Autodesk Fusion 360 part; units mm, degrees
sketch "Sketch1" plane through (0, 0, 0) normal (0, 0, 1) x (1, 0, 0)
  line L0 (0, 0) -> (-89.8767, -4.7102)
  line L1 (0, 0) -> (90, 0) construction
  line L2 (0, 0) -> (0, 36)
  line L3 (0, 36) -> (-89.8767, 40.7102)
  line L4 (0, 36) -> (90, 36) construction
  line L5 (-89.8767, 40.7102) -> (-89.8767, -4.7102)
  dimension "d1" = 177
  dimension "d2" = 90
  dimension "d3" = 36
  dimension "d4" = 177
  dimension "d5" = 90
extrude "Extrude1" add sketch "Sketch1" along normal blind 6 draft 45
fillet "Fillet1" radius 10 2 edges at (3, -2.8469, 3) (3, 38.8469, 3)
sketch "Sketch2" plane through (0, 0, 0) normal (0, 0, -1) x (1, 0, 0)
  ellipse E0 centre (-14.1421, -22.5796) end of major axis (-1.7883, -34.3029) minor radius 10 (-6.701, -36.3512) -> (0, -29.2898) ccw
  line L0 (0, -29.2898) -> (0, -6.7102)
  ellipse E1 centre (-14.1421, -13.4204) end of major axis (-1.7883, -1.6971) minor radius 10 (0, -6.7102) -> (-6.701, 0.3512) ccw
  line L1 (-6.701, 0.3512) -> (-89.8767, 4.7102)
  line L2 (-89.8767, 4.7102) -> (-89.8767, -40.7102)
  line L3 (-89.8767, -40.7102) -> (-6.701, -36.3512)
  line L4 (-89.8767, 4.7102) -> (-89.8767, -18) construction
  line L5 (-89.8767, -18) -> (-45.8767, -18) construction
  line L6 (-6.8767, -33.25) -> (-84.8767, -33.25)
  line L7 (-84.8767, -33.25) -> (-84.8767, -2.75)
  line L8 (-84.8767, -2.75) -> (-6.8767, -2.75)
  line L9 (-6.8767, -2.75) -> (-6.8767, -33.25)
  line L10 (-6.8767, -33.25) -> (-84.8767, -2.75) construction
  line L11 (-84.8767, -33.25) -> (-6.8767, -2.75) construction
  point P0 (-45.8767, -18)
  dimension "d10" = 22.7102
  dimension "d11" = 44
  dimension "d12" = 78
  dimension "d13" = 30.5
extrude "Extrude2" cut sketch "Sketch2" against normal blind 1.5 contours L6 L7 L8 L9
sketch "Sketch3" plane through (0, 0, 0) normal (0, 0, -1) x (1, 0, 0)
  line L0 (-84.8767, -33.25) -> (-84.8767, -2.75)
  line L1 (-84.8767, -2.75) -> (-6.8767, -2.75)
  line L2 (-6.8767, -2.75) -> (-6.8767, -33.25)
  line L3 (-6.8767, -33.25) -> (-84.8767, -33.25)
  ellipse E0 centre (-14.1421, -22.5796) end of major axis (-1.7883, -34.3029) minor radius 10 (-6.701, -36.3512) -> (0, -29.2898) ccw
  line L4 (0, -29.2898) -> (0, -6.7102)
  ellipse E1 centre (-14.1421, -13.4204) end of major axis (-1.7883, -1.6971) minor radius 10 (0, -6.7102) -> (-6.701, 0.3512) ccw
  line L5 (-6.701, 0.3512) -> (-89.8767, 4.7102)
  line L6 (-89.8767, 4.7102) -> (-89.8767, -40.7102)
  line L7 (-89.8767, -40.7102) -> (-6.701, -36.3512)
sketch "Sketch4" plane through (0, 0, 0) normal (0, 0, -1) x (1, 0, 0)
  line L0 (-85, -15) -> (-85, 16.158)
  line L1 (-85, 16.158) -> (-101.3363, 16.158)
  line L2 (-101.3363, 16.158) -> (-101.3363, -48.0286)
  line L3 (-101.3363, -48.0286) -> (-85, -48.0286)
  line L4 (-85, -48.0286) -> (-85, -15)
extrude "Extrude3" cut sketch "Sketch4" against normal blind 15
sketch "Sketch5" plane through (-85, 0, 0) normal (-1, 0, 0) x (0, -1, 0)
  line L0 (4.4547, 0) -> (10.4629, 6)
  line L1 (10.4629, 6) -> (-46.4629, 6)
  line L2 (-46.4629, 6) -> (-40.4547, 0)
  line L3 (-40.4547, 0) -> (4.4547, 0)
  line L4 (-46.4629, 6) -> (-18, 6)
  line L5 (10.4629, 6) -> (-18, 6)
  circle A0 centre (-18, 6) radius 3
  dimension "d18" = 28.4629
  dimension "d19" = 6
extrude "Extrude4" cut sketch "Sketch5" against normal blind 100 contours L1 L4 L5 A0 picked at (-19.9888, 5.851)
chamfer "Chamfer1" distance 0.5 angle 45 10 edges at (-42.8505, -8.2539, 6) (6, 8.0082, 6) (4.2117, -3.9967, 6) (3, 18, 3) (6, 27.9918, 6) (-42.8505, 44.2539, 6) (4.2117, 39.9967, 6) (-85, 33.7314, 6) (-85, 18, 3) (-85, 2.2686, 6)
chamfer "Chamfer2" distance 0.5 angle 45 10 edges at (-1.7883, 34.3029, 0) (-45.8505, 38.4029, 0) (-45.8505, -2.4029, 0) (-1.7883, 1.6971, 0) (0, 18, 0) (-85, -7.2084, 2.75) (-85, 43.2084, 2.75) (-45.8767, 33.25, 0) (-6.8767, 18, 0) (-45.8767, 2.75, 0)
sketch "Sketch6" plane through (0, 0, 6) normal (0, 0, 1) x (-1, 0, 0)
  spline S0 degree 3 poles (-5.2935, -15) (-5.3627, -14.9531) (-5.4315, -14.9058) (-5.5, -14.8582) knots 0 0 0 0 0.025071 0.025071 0.025071 0.025071
  line L0 (-5.2935, -15) -> (84.5, -15)
  line L1 (84.5, -15) -> (84.5, 9.936)
  line L2 (84.5, 9.936) -> (1.0622, 5.5632)
  line L3 (0.7272, 5.5457) -> (1.0622, 5.5632)
  spline S1 degree 3 poles (-5.5, -1.0164) (-5.5, -0.8241) (-5.4943, -0.6349) (-5.4197, 0.5909) (-5.1793, 1.5237) (-4.5302, 2.8177) (-4.2188, 3.2629) (-3.849, 3.6526) (-3.4792, 4.0422) (-3.051, 4.3765) (-1.7926, 5.0924) (-0.8738, 5.3813) (0.3465, 5.52) (0.5351, 5.5356) (0.7272, 5.5457) knots -0.508354 -0.508354 -0.508354 -0.508354 -0.45799 -0.45799 -0.17615 -0.17615 0 0 0 0.17615 0.17615 0.45799 0.45799 0.508354 0.508354 0.508354 0.508354
  line L4 (-5.5, -1.3519) -> (-5.5, -1.0164)
  line L5 (-5.5, -1.3519) -> (-5.5, -14.8582)
  line L6 (82, -17.9581) -> (47, -17.9581) construction
  line L7 (74.5, -7.9581) -> (19.5, -7.9581) construction
  line L8 (19.5, -7.9581) -> (19.5, -27.9581) construction
  line L9 (19.5, -27.9581) -> (74.5, -27.9581) construction
  line L10 (74.5, -27.9581) -> (74.5, -7.9581) construction
  line L11 (74.5, -7.9581) -> (19.5, -27.9581) construction
  line L12 (19.5, -7.9581) -> (74.5, -27.9581) construction
  point P0 (47, -17.9581)
  dimension "d24" = 35
  dimension "d25" = 55
  dimension "d26" = 20
hole "Hole1" at (-19.5, 27.9581, 6) at (-19.5, 7.9581, 6) at (-74.5, 27.9581, 6) at (-74.5, 7.9581, 6) direction (0, 0, -1) diameter 3 depth 10 tip angle 118 countersink diameter 6 countersink angle 90
Source: CAD feature listing. Evaluate the final solid. Frame: model axes, mm. Give positions to 0.01 mm unless a question says otherwise; leave off trailing zeros. Order: outer loops, then holes, each group sorted by start corner. A loop starts at its lowest first (then second) coordinate and runs counter-clockwise, first axis right, second up.
(1) Section query C-C (x = -44.5). Return the cut outline in (y, z).
(2) Section query B-B (x = -59.5). Return the cut outline in (y, z).
(3) Section query A-A (x = -19.5). Return the cut outline in (y, z).
(4) Material intervals for line 1 along Y through (x, z) = (-19.5, 3.45); line 2 along Y through (x, z) = (-74.5, 2.3); line 3 along Y through (x, z) = (-39, 5.25), sorted ascending.
(5) Pull-direction query (Y, two-part tool) for faces 1 (the face through (-21, 28, 3)), 2 (the face through (-43.453, -7.857, 5.826)), 3 (the face through (-84.75, 42.9, 2.81)); classes: +Y half, -Y half, draft (parallel to the pull), parting line (faces both ways), or undercut.
(6) Contact query for flat-ended pins moving along their axis: P1, Ø3.5, axis at x = -19.5, y = 7.96, coming from the +Z side; P2, Ø4, axis at x = -74.5, y = 7.96, coming from the -Z side; P3, Ø1, axis at x = -11.5, z = 5, coming from the +Y side. Output: stop coordinate, or through.
Outcome:
1. outline: (-7.99, 5.65) - (-2.69, 0.35) - (-1.83, 0) - (2.25, 0) - (2.75, 0.5) - (2.75, 1.5) - (33.25, 1.5) - (33.25, 0.5) - (33.75, 0) - (37.83, 0) - (38.69, 0.35) - (43.99, 5.65) - (43.84, 6) - (21, 6) arc R3 cw to (15, 6) - (-7.84, 6) - close
2. outline: (-8.77, 5.65) - (-3.47, 0.35) - (-2.62, 0) - (2.25, 0) - (2.75, 0.5) - (2.75, 1.5) - (33.25, 1.5) - (33.25, 0.5) - (33.75, 0) - (38.62, 0) - (39.47, 0.35) - (44.77, 5.65) - (44.63, 6) - (21, 6) arc R3 cw to (15, 6) - (-8.63, 6) - close
3. outline: (-6.68, 5.65) - (-1.38, 0.35) - (-0.52, 0) - (2.25, 0) - (2.75, 0.5) - (2.75, 1.5) - (6.46, 1.5) - (6.46, 4.5) - (4.96, 6) - (-6.53, 6) - close; (9.46, 1.5) - (26.46, 1.5) - (26.46, 4.5) - (24.96, 6) - (21, 6) arc R3 cw to (15, 6) - (10.96, 6) - (9.46, 4.5) - close; (29.46, 1.5) - (33.25, 1.5) - (33.25, 0.5) - (33.75, 0) - (36.52, 0) - (37.38, 0.35) - (42.68, 5.65) - (42.53, 6) - (30.96, 6) - (29.46, 4.5) - close
4. line 1: y = -4.48 to 6.46, 9.46 to 16.42, 19.58 to 26.46, 29.46 to 40.48
4. line 2: y = -6.21 to 6.46, 9.46 to 26.46, 29.46 to 42.21
4. line 3: y = -7.3 to 15.1, 20.9 to 43.3
5. face 1: undercut
5. face 2: -Y half
5. face 3: +Y half
6. P1: stops at z = 4.75
6. P2: stops at z = 1.5
6. P3: stops at y = 42.11
